Design review of the part built by this model. Coordinates are the model's own, in mm. A direction names the side the tool comes from. Coordinates: 2 decimals unless noted, no trailing zeros. Loops run counter-clockwise (first coordinate to the right, second up) from the corner with the lowest first, then second, coordinate; pieces in that order, holes last. Notation, with made-up numbers: M -30,72 L -13,72 A21 ccw -13,95 Z; hole C -10,-22 d7. An arc over 180 degrees is marked long. Put each result on its own line as item: value. Start each with the question number.
(1) For probe 1 along Z at (x, y) = (0, 0.4) (3 decimals); probe 2 along Z at (x, y) = (0, 6.25) (3 decimals); probe 3 along Y at (x, z) = (-1.5, -4.5), list the stretches that pass through material, from the lowest coordinate up. Write a range as [from, to].
(2) Take a section at D-D, the plane z = 11.25. Give the boundary of the cut face in (x, y).
(3) Clearance check with flat-ended pins moving along their axes: pin 1 (1.5 mm diameter, centred on x = -1.5, y = 2, fed in from -Z); pin 2 (5 mm diameter, centred on x = 4.5, y = 9, fed in from +Z); pin 3 (4 mm diameter, centred on x = 3, y = 5.5, fed in from +Z). State where each tip first meets the part, or that it passes through.
(4) Take a section at A-A, the plane x = 0. Give the boundary of the cut face in (y, z) (3 decimals), then the cut area to 3 significant figures.
(5) For faces 5 (the flat face through (-2.392, 0.431, 7.44)), 6 (the flat face through (2.42, 0.43, 7.37)), 7 (the cylindrical face through (-0.61, 6.27, 14.62)), list the 3-axis set-ups (+Z, -Z, +X, -X, +Y, -Y) from which the entire face can be reached by the end or side of a thin tool; tool diameter is ignored.
(6) Take a section at B-B, the plane z = 0. Give the boundary of the cut face in (x, y) (3 decimals).
(7) Take a section at C-C, the plane y = 2.75. Give the boundary of the cut face in (x, z) (3 decimals), then the cut area to 3 significant figures.
(8) The part is to be moulded in two halves that separate along Z. For faces 1 (the cylindrical face through (0.69, 0.42, 3.1)), 2 (the flat face through (1.2, 12.37, 12.5)), 3 (the cylindrical face through (-0.15, 6.1, 10.73)), 4 (the cylindrical face through (0.21, 0.419, -5.956)), say which applies: +Z half, -Z half, draft (parallel to the pull), parting line (faces both ways), or undercut.
```python
from build123d import *

# Parameters (mm, degrees)
SKETCH1_R                       = 5.96
BOSS_EXTRUDE1_DEPTH             = 0.85
F_1_4_0_25_DIAMETER_HOLE1_D     = 6.35
F_1_4_0_25_DIAMETER_HOLE1_DEPTH = 0.85
SKETCH5_R                       = 2.81
SKETCH5_R_2                     = 1.155
BOSS_EXTRUDE2_DEPTH             = 11.52
BOSS_EXTRUDE2_DEPTH_BACK        = 0.85
BOSS_EXTRUDE3_DEPTH             = 0.85
SKETCH9_R                       = 1.155
CUT_EXTRUDE1_DEPTH              = 1.85


with BuildPart() as part:
    # Sketch1 → Boss-Extrude1 (new body)
    with BuildSketch(Plane(origin=(0, 0, 0), x_dir=(1, 0, 0), z_dir=(0, 1, 0))):
        Circle(SKETCH1_R)
    extrude(amount=BOSS_EXTRUDE1_DEPTH)

    # 1/4 (0.25) Diameter Hole1
    with Locations(Plane(origin=(0, 0.85, 0), x_dir=(1, 0, 0), z_dir=(0, 1, 0))):
        with Locations((0, 0)):
            Hole(F_1_4_0_25_DIAMETER_HOLE1_D / 2, depth=F_1_4_0_25_DIAMETER_HOLE1_DEPTH)



with BuildPart() as body_2:
    # Sketch5 → Boss-Extrude2 (new body, two sides)
    with BuildSketch(Plane(origin=(0, 0.85, 0), x_dir=(1, 0, 0), z_dir=(0, 1, 0))) as boss_extrude2_sk:
        with Locations((0, -11.875)):
            Circle(SKETCH5_R)
        with Locations((0, -11.875)):
            Circle(SKETCH5_R_2, mode=Mode.SUBTRACT)
    extrude(amount=BOSS_EXTRUDE2_DEPTH)
    extrude(boss_extrude2_sk.sketch, amount=-BOSS_EXTRUDE2_DEPTH_BACK)


with BuildPart() as part_1:
    add(part.part)

    add(body_2.part)  # Boss-Extrude3 merges body 2
    # Sketch6 → Boss-Extrude3 (add)
    with BuildSketch(Plane(origin=(0, 0.85, 0), x_dir=(1, 0, 0), z_dir=(0, 1, 0))):
        Polygon((-1.155, -11.875), (-3.036993485, -5.128183945), (3.04994253, -5.120493195), (1.155, -11.875), align=None)
    extrude(amount=-BOSS_EXTRUDE3_DEPTH)

    # Sketch9 → Cut-Extrude1 (cut, through all)
    with BuildSketch(Plane(origin=(0, 0.85, 0), x_dir=(1, 0, 0), z_dir=(0, 1, 0))):
        with Locations((0, -11.875)):
            Circle(SKETCH9_R)
    extrude(amount=-CUT_EXTRUDE1_DEPTH, mode=Mode.SUBTRACT)


solid = part_1.part
```
Computed values:
1. probe 1: z = [-5.96, -3.175], [3.175, 10.72], [13.03, 14.685]
1. probe 2: z = [9.065, 10.72], [13.03, 14.685]
1. probe 3: y = [0, 0.85]
2. outline: M -2.74,0 L -0.97,0 L -0.97,12.37 L -2.74,12.37 Z; M 0.97,0 L 2.74,0 L 2.74,12.37 L 0.97,12.37 Z
3. pin 1: stops at z = 9.17
3. pin 2: stops at z = 13.85
3. pin 3: stops at z = 14.5
4. outline: M 0,-5.96 L 0.85,-5.96 L 0.85,-3.175 L 0,-3.175 Z; M 0,3.175 L 0.85,3.175 L 0.85,9.065 L 12.37,9.065 L 12.37,10.72 L 0,10.72 Z; M 0,13.03 L 12.37,13.03 L 12.37,14.685 L 0,14.685 Z
4. area: 48.3 mm^2
5. face 5: -X, +Y, -Y
5. face 6: +X, +Y, -Y
5. face 7: +Y
6. outline: M -5.96,0 L -3.175,0 L -3.175,0.85 L -5.96,0.85 Z; M 3.175,0 L 5.96,0 L 5.96,0.85 L 3.175,0.85 Z
7. outline: C 0,11.875 d5.62; hole C 0,11.875 d2.31
7. area: 20.6 mm^2
8. face 1: undercut
8. face 2: draft
8. face 3: undercut
8. face 4: parting line
